Work out the finished part from the listing and answer in its coordinate system (mm). A direction names the side the tool comes from. Coordinates: 2 decimals unless noted, no trailing zeros. Order: outer loops, then holes, each group sorted by start corner. A loop starts at its lowest first (then second) coordinate and runs counter-clockwise, first axis right, second up. Notation, with made-up numbers: M -25.5,15.25 L 23.5,15.25 A29 ccw 23.5,38.25 Z; hole C -32,71.25 d8. An arc over 180 degrees is marked long. Use a Markdown table: item, result.
from build123d import *

# Parameters (mm, degrees)
SKETCH1_R           = 1.5
SKETCH1_W           = 3.5
SKETCH1_H           = 7
BOSS_EXTRUDE1_DEPTH = 3


with BuildPart() as part:
    # Sketch1 → Boss-Extrude1 (new body)
    with BuildSketch(Plane.XY):
        with BuildLine():
            Line((4, 0), (207, 0))
            ThreePointArc((207, 0), (209.828427125, 1.171572875), (211, 4))
            Line((211, 4), (211, 44.117670932))
            ThreePointArc((211, 44.117670932), (209.828427125, 46.946098057), (207, 48.117670932))
            Line((207, 48.117670932), (4, 48.117670932))
            ThreePointArc((4, 48.117670932), (1.171572875, 46.946098057), (0, 44.117670932))
            Line((0, 44.117670932), (0, 4))
            ThreePointArc((0, 4), (1.171572875, 1.171572875), (4, 0))
        make_face()
        with Locations((32.5, 40.617670932)):
            Circle(SKETCH1_R, mode=Mode.SUBTRACT)
        with Locations((19.5, 7.5)):
            Circle(SKETCH1_R, mode=Mode.SUBTRACT)
        with Locations((60.5, 40.617670932)):
            Circle(SKETCH1_R, mode=Mode.SUBTRACT)
        with Locations((47.5, 7.5)):
            Circle(SKETCH1_R, mode=Mode.SUBTRACT)
        with Locations((98, 40.617670932)):
            Circle(SKETCH1_R, mode=Mode.SUBTRACT)
        with Locations((85, 7.5)):
            Circle(SKETCH1_R, mode=Mode.SUBTRACT)
        with Locations((126, 40.617670932)):
            Circle(SKETCH1_R, mode=Mode.SUBTRACT)
        with Locations((113, 7.5)):
            Circle(SKETCH1_R, mode=Mode.SUBTRACT)
        with Locations((8, 40.117670932)):
            Circle(SKETCH1_R, mode=Mode.SUBTRACT)
        with Locations((8, 8)):
            Circle(SKETCH1_R, mode=Mode.SUBTRACT)
        with Locations((203, 8)):
            Circle(SKETCH1_R, mode=Mode.SUBTRACT)
        with Locations((203, 40.117670932)):
            Circle(SKETCH1_R, mode=Mode.SUBTRACT)
        with Locations((163.5, 40.617670932)):
            Circle(SKETCH1_R, mode=Mode.SUBTRACT)
        with Locations((150.5, 7.5)):
            Circle(SKETCH1_R, mode=Mode.SUBTRACT)
        with Locations((191.5, 40.617670932)):
            Circle(SKETCH1_R, mode=Mode.SUBTRACT)
        with Locations((178.5, 7.5)):
            Circle(SKETCH1_R, mode=Mode.SUBTRACT)
        with BuildLine():
            Line((15, 15), (15, 33.117670932))
            ThreePointArc((15, 33.117670932), (26, 38.308835466), (37, 33.117670932))
            Line((37, 33.117670932), (37, 15))
            ThreePointArc((37, 15), (26, 9.808835466), (15, 15))
        make_face(mode=Mode.SUBTRACT)
        with BuildLine():
            Line((43, 15), (43, 33.117670932))
            ThreePointArc((43, 33.117670932), (54, 38.308835466), (65, 33.117670932))
            Line((65, 33.117670932), (65, 15))
            ThreePointArc((65, 15), (54, 9.808835466), (43, 15))
        make_face(mode=Mode.SUBTRACT)
        with BuildLine():
            Line((80.5, 15), (80.5, 33.117670932))
            ThreePointArc((80.5, 33.117670932), (91.5, 38.308835466), (102.5, 33.117670932))
            Line((102.5, 33.117670932), (102.5, 15))
            ThreePointArc((102.5, 15), (91.5, 9.808835466), (80.5, 15))
        make_face(mode=Mode.SUBTRACT)
        with Locations((72.75, 32.117670932)):
            Rectangle(SKETCH1_W, SKETCH1_H, mode=Mode.SUBTRACT)
        with Locations((72.75, 16)):
            Rectangle(SKETCH1_W, SKETCH1_H, mode=Mode.SUBTRACT)
        with BuildLine():
            Line((108.5, 15), (108.5, 33.117670932))
            ThreePointArc((108.5, 33.117670932), (119.5, 38.308835466), (130.5, 33.117670932))
            Line((130.5, 33.117670932), (130.5, 15))
            ThreePointArc((130.5, 15), (119.5, 9.808835466), (108.5, 15))
        make_face(mode=Mode.SUBTRACT)
        with BuildLine():
            Line((146, 15), (146, 33.117670932))
            ThreePointArc((146, 33.117670932), (157, 38.308835466), (168, 33.117670932))
            Line((168, 33.117670932), (168, 15))
            ThreePointArc((168, 15), (157, 9.808835466), (146, 15))
        make_face(mode=Mode.SUBTRACT)
        with Locations((138.25, 32.117670932)):
            Rectangle(SKETCH1_W, SKETCH1_H, mode=Mode.SUBTRACT)
        with Locations((138.25, 16)):
            Rectangle(SKETCH1_W, SKETCH1_H, mode=Mode.SUBTRACT)
        with BuildLine():
            Line((174, 15), (174, 33.117670932))
            ThreePointArc((174, 33.117670932), (185, 38.308835466), (196, 33.117670932))
            Line((196, 33.117670932), (196, 15))
            ThreePointArc((196, 15), (185, 9.808835466), (174, 15))
        make_face(mode=Mode.SUBTRACT)
    extrude(amount=BOSS_EXTRUDE1_DEPTH)


solid = part.part
1. Section B-B on x = 119 is taken. Determine the outline of the cut face in (y, z), then the cut area to 3 significant figures.
Answers below:
| item | result |
|---|---|
| outline | M 0,0 L 9.82,0 L 9.82,3 L 0,3 Z; M 38.3,0 L 48.12,0 L 48.12,3 L 38.3,3 Z |
| area | 58.9 mm² |
2. Find the intervals of material crossed by probe 1 along Y at (x, z) = (203, 0.95); probe 2 along Y at (x, z) = (60.5, 1.6); probe 3 along Y at (x, z) = (100, 2.3), in increasing order.
Answers below:
| item | result |
|---|---|
| probe 1 | 0 to 6.5, 9.5 to 38.62, 41.62 to 48.12 |
| probe 2 | 0 to 11.38, 36.74 to 39.12, 42.12 to 48.12 |
| probe 3 | 0 to 12.62, 35.5 to 48.12 |
3. For faces 4 (the face through (91.68, 9.81, 1.48)), 5 (the face through (104, 24, 0)), determine the directions among +Z, -Z, +X, -X, +Y, -Y from which every point of the face is accessible in a straight line to the end or side of a thin tool.
Answers below:
| item | result |
|---|---|
| face 4 | +Z, -Z |
| face 5 | -Z, +X, -X, +Y, -Y |
4. Section A-A on y = 23.5 is taken. Determine the outline of the cut face in (x, z).
Answers below:
| item | result |
|---|---|
| outline | M 0,0 L 15,0 L 15,3 L 0,3 Z; M 37,0 L 43,0 L 43,3 L 37,3 Z; M 65,0 L 80.5,0 L 80.5,3 L 65,3 Z; M 102.5,0 L 108.5,0 L 108.5,3 L 102.5,3 Z; M 130.5,0 L 146,0 L 146,3 L 130.5,3 Z; M 168,0 L 174,0 L 174,3 L 168,3 Z; M 196,0 L 211,0 L 211,3 L 196,3 Z |
5. Section C-C on z = 1.6 is taken. Give the number of separate pieces and of enclosed holes in the cut face, then the cut area to 3 significant figures.
Answers below:
| item | result |
|---|---|
| separate pieces | 1 |
| enclosed holes | 26 |
| area | 6,580 mm² |
6. For a pull along Y with two mould halves and no side action, classify faces 1 (the face through (1.203, 46.977, 1.479)), 2 (the face through (104, 24, 3)), 3 (the face through (119.68, 9.81, 1.48)) as +Y half, -Y half, draft (parallel to the pull), parting line (faces both ways), or undercut.
Answers below:
| item | result |
|---|---|
| face 1 | +Y half |
| face 2 | draft |
| face 3 | undercut |
7. A flat-ended cylindrical pin translates along its axis: P1, Ø1.8, axis at x = 32.5, y = 40.62, coming from the -Z side. Find the tip coordinate at first contact, or state that the pin passes through.
Answers below:
| item | result |
|---|---|
| P1 | through |
